Geometry check sheet. Reference: drawing and pictorial views, mm from the part's lowest x, y, z. Round coordinates to 2 decimals unless told otherwise and drop trailing zeros. Loops run counter-clockwise (first coordinate to the right, second up) from the corner with the lowest first, then second, coordinate; pieces in that order, holes last. Notation, with made-up numbers: (-34, -2.5) - (19, -2.5) arc R8 ccw to (19, 10.5) - close; hole circle Ø6 at (-19, 89.5). An arc over 180 degrees is marked (long way). Put each result on its own line as item: value. Start each with the question number.
Item 1: Section check B-B, the plane y = 19. Record the cut outline in (x, z).
Item 2: Section check A-A, the plane z = 1.55. Give the number of separate pieces and of enclosed holes in the cut face, and give its area (3 significant figures).
Item 3: Section check C-C, the plane x = 28.5. Record the cut outline in (y, z), and give its area (3 significant figures).
Item 4: Material ranges on line 1 along Y through (x, z) = (94, 1.05); line 2 along Y through (x, z) = (4, 0.55); line 3 along X through (y, z) = (2.5, 0.9) (1 decimal), recorded low to high.
Item 5: Gauge pin test, flat ends, axial feed: pin 1 Ø1 at (x, z) = (60.5, 1) entering from -Y; pin 2 Ø1 at (y, z) = (4.5, 1.5) entering from -X; pin 3 Ø1 at (y, z) = (19.5, 1) entering from -X. Record the tip position at first contact, or that the pin passes through.
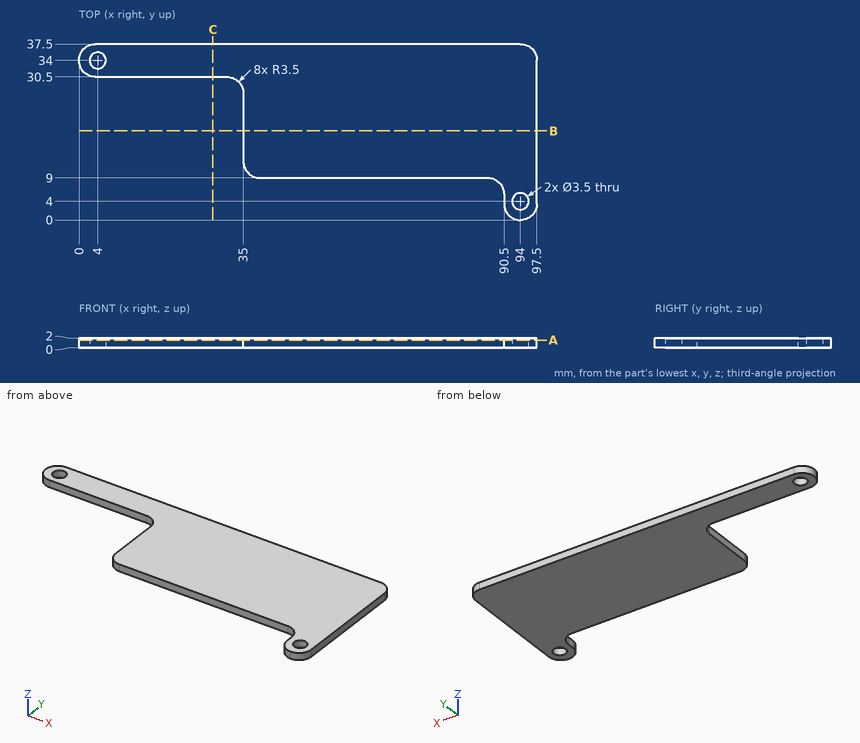
Check result:
1. outline: (35, 0) - (97.5, 0) - (97.5, 2) - (35, 2) - close
2. separate pieces: 1
2. enclosed holes: 2
2. area: 2,060 mm²
3. outline: (30.5, 0) - (37.5, 0) - (37.5, 2) - (30.5, 2) - close
3. area: 14.0 mm²
4. line 1: 0 to 2.25, 5.75 to 37.5
4. line 2: 30.5 to 32.25, 35.75 to 37.5
4. line 3: 90.6 to 93.1, 94.9 to 97.4
5. pin 1: y = 9
5. pin 2: x = 90.5
5. pin 3: x = 35
